```python
from build123d import *

# Parameters (mm, degrees)
ESQUISSE1_R        = 4
ESQUISSE1_R_2      = 2
BOSS_EXTRU_1_DEPTH = 15
ESQUISSE2_R        = 5
ESQUISSE2_R_2      = 2
BOSS_EXTRU_2_DEPTH = 1.25
ESQUISSE3_R        = 5
ESQUISSE3_R_2      = 2
BOSS_EXTRU_3_DEPTH = 2.5
BOSS_EXTRU_5_START = -1.25
ESQUISSE5_R        = 5
ESQUISSE5_R_2      = 2
BOSS_EXTRU_5_DEPTH = 1.25


with BuildPart() as part:
    # Esquisse1 → Boss.-Extru.1 (new body)
    with BuildSketch(Plane(origin=(0, 0, 0), x_dir=(1, 0, 0), z_dir=(0, 1, 0))):
        with Locations(Location((0, 0, 0), (0, 0, 270))):
            Circle(ESQUISSE1_R)
        with Locations(Location((0, 0, 0), (0, 0, 270))):
            Circle(ESQUISSE1_R_2, mode=Mode.SUBTRACT)
    extrude(amount=BOSS_EXTRU_1_DEPTH)

    # Esquisse2 → Boss.-Extru.2 (add)
    with BuildSketch(Plane(origin=(0, 0, 0), x_dir=(1, 0, 0), z_dir=(0, 1, 0))):
        with Locations(Location((0, 0, 0), (0, 0, 270))):
            Circle(ESQUISSE2_R)
        with Locations(Location((0, 0, 0), (0, 0, 270))):
            Circle(ESQUISSE2_R_2, mode=Mode.SUBTRACT)
    extrude(amount=BOSS_EXTRU_2_DEPTH)

    # Esquisse3 → Boss.-Extru.3 (add)
    with BuildSketch(Plane(origin=(0, 6.25, 0), x_dir=(1, 0, 0), z_dir=(0, 1, 0))):
        with Locations(Location((0, 0, 0), (0, 0, 270))):
            Circle(ESQUISSE3_R)
        with Locations(Location((0, 0, 0), (0, 0, 270))):
            Circle(ESQUISSE3_R_2, mode=Mode.SUBTRACT)
    extrude(amount=BOSS_EXTRU_3_DEPTH)

    # Esquisse5 → Boss.-Extru.5 (add)
    with BuildSketch(Plane(origin=(0, 15, 0), x_dir=(1, 0, 0), z_dir=(0, 1, 0)).offset(BOSS_EXTRU_5_START)):
        with Locations(Location((0, 0, 0), (0, 0, 270))):
            Circle(ESQUISSE5_R)
        with Locations(Location((0, 0, 0), (0, 0, 270))):
            Circle(ESQUISSE5_R_2, mode=Mode.SUBTRACT)
    extrude(amount=BOSS_EXTRU_5_DEPTH)


solid = part.part
```
Geometry check sheet. Reference: the model listing, model coordinates, mm. A direction names the side the tool comes from. Coordinates: 2 decimals unless noted, no trailing zeros. Write each loop counter-clockwise with the first axis right and the second up, starting at its lowest first coordinate (ties: lowest second). Pieces come first, ordered by that corner, then holes. Notation, with made-up numbers: M 21.5,46.5 L 75.5,46.5 A9 cw 75.5,57.5 Z; hole C 11.5,55 d7. An arc over 180 degrees is marked long. Answer as a JSON object with one key per item and string values.
1. Section check B-B, the plane x = 0. Enter the section's corners in (y, z), plus the area to 3 significant figures.
Answers below:
{"outline": "M 0,-5 L 1.25,-5 L 1.25,-4 L 6.25,-4 L 6.25,-5 L 8.75,-5 L 8.75,-4 L 13.75,-4 L 13.75,-5 L 15,-5 L 15,-2 L 0,-2 Z; M 0,2 L 15,2 L 15,5 L 13.75,5 L 13.75,4 L 8.75,4 L 8.75,5 L 6.25,5 L 6.25,4 L 1.25,4 L 1.25,5 L 0,5 Z", "area": "70.0 mm²"}
2. Scan lines: L1, parallel to Y at x = 1.25, z = 4.25; L2, parallel to X at y = 5.75, z = 0; L3, parallel to X at y = 6.75, z = 0. Record each from-to range of solid material in increasing order.
Answers below:
{"L1": "y = 0 to 1.25, 6.25 to 8.75, 13.75 to 15", "L2": "x = -4 to -2, 2 to 4", "L3": "x = -5 to -2, 2 to 5"}
3. Go/stop test with flat-tipped pins: pin 1 Ø1 at (y, z) = (1.5, 3) entering from +X; pin 2 Ø3.5 at (x, z) = (0, 0) entering from -Y; pin 3 Ø6 at (y, z) = (13, -4) entering from -X; pin 4 Ø1 at (x, y) = (4, 7) entering from -Z. Record where each tip stops, or that it passes through.
Answers below:
{"pin 1": "stops at x = 4.29", "pin 2": "passes through", "pin 3": "stops at x = -4.88", "pin 4": "stops at z = -3.57"}
4. Section check D-D, the plane y = 6.5. Enter the section's corners in (x, z).
Answers below:
{"outline": "C 0,0 d10; hole C 0,0 d4"}
5. Draft check along Y on faces 3 (the flat face through (0.1, 15, 2.2)), 4 (the cylindrical face through (-2, 7, 0)), 5 (the flat face through (0.1, 0, 2.2)), 6 (the cylindrical face through (-3.905, 3.715, -0.867)). Enter one of: released by +Y, released by -Y, zero draft, split by the parting line, or undercut.
Answers below:
{"face 3": "released by +Y", "face 4": "zero draft", "face 5": "released by -Y", "face 6": "undercut"}
6. Section check C-C, the plane z = 3.5. Enter the section's corners in (x, y).
Answers below:
{"outline": "M -3.57,0 L 3.57,0 L 3.57,1.25 L 1.94,1.25 L 1.94,6.25 L 3.57,6.25 L 3.57,8.75 L 1.94,8.75 L 1.94,13.75 L 3.57,13.75 L 3.57,15 L -3.57,15 L -3.57,13.75 L -1.94,13.75 L -1.94,8.75 L -3.57,8.75 L -3.57,6.25 L -1.94,6.25 L -1.94,1.25 L -3.57,1.25 Z"}
7. Tool access check on faces 1 (the cylindrical face through (-4.88, 0.62, -1.08)), 2 (the cylindrical face through (-3.905, 11.215, -0.867)). Record the directions out of +Z, -Z, +X, -X, +Y, -Y that give a thin tool (end or side, any length) a straight path to the whole face; none if there is none.
Answers below:
{"face 1": "+Y, -Y", "face 2": "none"}
8. Section check A-A, the plane z = 0. Enter the section's corners in (x, y).
Answers below:
{"outline": "M -5,0 L -2,0 L -2,15 L -5,15 L -5,13.75 L -4,13.75 L -4,8.75 L -5,8.75 L -5,6.25 L -4,6.25 L -4,1.25 L -5,1.25 Z; M 2,0 L 5,0 L 5,1.25 L 4,1.25 L 4,6.25 L 5,6.25 L 5,8.75 L 4,8.75 L 4,13.75 L 5,13.75 L 5,15 L 2,15 Z"}
